Source: three-view drawing plus pictorial views. Frame: mm from the lowest corner of the part. A direction names the side the tool comes from. Coordinates: 2 decimals unless noted, no trailing zeros. Loops run counter-clockwise (first coordinate to the right, second up) from the corner with the lowest first, then second, coordinate; pieces in that order, holes last.
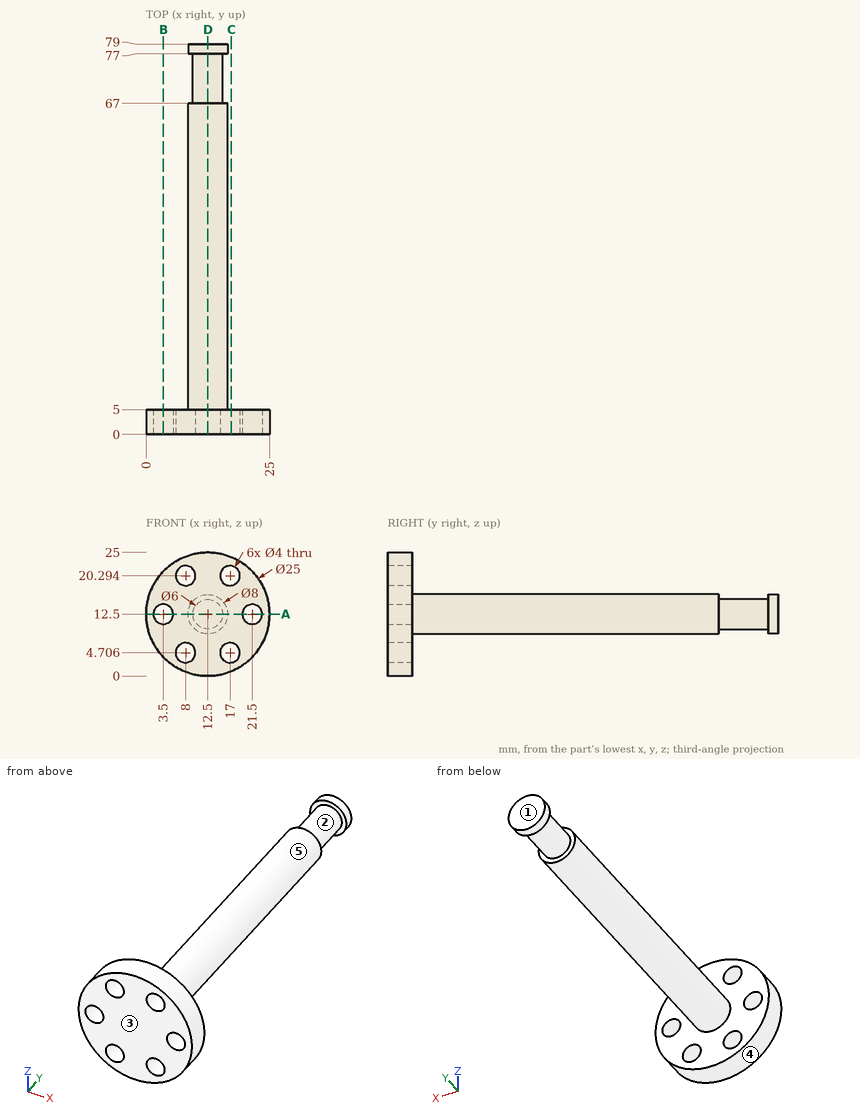
Q1. Section query A-A on z = 12.5. Return the cut outline in (x, y).
Q2. Section query B-B on x = 3.5. Return the cut outline in (y, z) (1 decimal).
Q3. Draft query along Y for the marked faces 1, 2 and 3. Return one class per face: released by +Y, released by -Y, zero draft, split by the parting line, or undercut.
Q4. First-contact query: pin 1 Ø4 at (y, z) = (62.5, 12) entering from -X; pin 2 Ø2 at (x, y) = (14, 39) entering from +Z; pin 3 Ø6.5 at (x, z) = (8, 20.29) entering from -Y; pin 4 Ø4 at (x, z) = (7, 5) entering from +Y. Flat tips, straight axial feed; report the tip coordinate or a pass-through.
Q5. Material intervals for line 1 along X through (y, z) = (4, 12.5); line 2 along Y through (x, z) = (13.5, 17.25); line 3 along Z through (x, y) = (3.5, 3.7) (1 decimal), sorted ascending.
Q6. Section query D-D on x = 12.5. Return the cut outline in (y, z), then the cut area to 3 significant figures.
Q7. Reachability of the marked faces 4 and 5 from +Z, -Z, +X, -X, +Y, -Y: full face, straight path, thin tool, end or side. Return the list, or none.
Q8. Section query C-C on x = 17.25. Return the cut outline in (y, z).
Resolved:
1. outline: (0, 0) - (1.5, 0) - (1.5, 5) - (0, 5) - close; (5.5, 0) - (19.5, 0) - (19.5, 5) - (16.5, 5) - (16.5, 67) - (15.5, 67) - (15.5, 77) - (16.5, 77) - (16.5, 79) - (8.5, 79) - (8.5, 77) - (9.5, 77) - (9.5, 67) - (8.5, 67) - (8.5, 5) - (5.5, 5) - close; (23.5, 0) - (25, 0) - (25, 5) - (23.5, 5) - close
2. outline: (0, 3.8) - (5, 3.8) - (5, 10.5) - (0, 10.5) - close; (0, 14.5) - (5, 14.5) - (5, 21.2) - (0, 21.2) - close
3. face 1: released by +Y
3. face 2: undercut
3. face 3: released by -Y
4. pin 1: stops at x = 8.5
4. pin 2: stops at z = 16.47
4. pin 3: stops at y = 0
4. pin 4: stops at y = 5
5. line 1: x = 0 to 1.5, 5.5 to 19.5, 23.5 to 25
5. line 2: y = 0 to 5
5. line 3: z = 3.8 to 10.5, 14.5 to 21.2
6. outline: (0, 0) - (5, 0) - (5, 8.5) - (67, 8.5) - (67, 9.5) - (77, 9.5) - (77, 8.5) - (79, 8.5) - (79, 16.5) - (77, 16.5) - (77, 15.5) - (67, 15.5) - (67, 16.5) - (5, 16.5) - (5, 25) - (0, 25) - close
6. area: 697 mm2
7. face 4: +Y, -Y
7. face 5: +Y
8. outline: (0, 0.94) - (5, 0.94) - (5, 2.72) - (0, 2.72) - close; (0, 6.69) - (5, 6.69) - (5, 18.31) - (0, 18.31) - close; (0, 22.28) - (5, 22.28) - (5, 24.06) - (0, 24.06) - close
